The listing builds one solid part. Answer for the finished solid, in the listing's coordinates (mm). Face numbers are marked on the shaded views. A direction names the side the tool comes from. Coordinates: 2 decimals unless noted, no trailing zeros. Order: outer loops, then holes, each group sorted by start corner. A loop starts at its lowest first (then second) coordinate and runs counter-clockwise, first axis right, second up. Notation, with made-up numbers: (52.25, -4.5) -> (94.25, -4.5) arc R23 cw to (94.25, 29.5) -> close; hole circle Ø3 at (-28.5, 26.25). An arc over 180 degrees is marked (long way). Return JSON: item names as keys, results as strings.
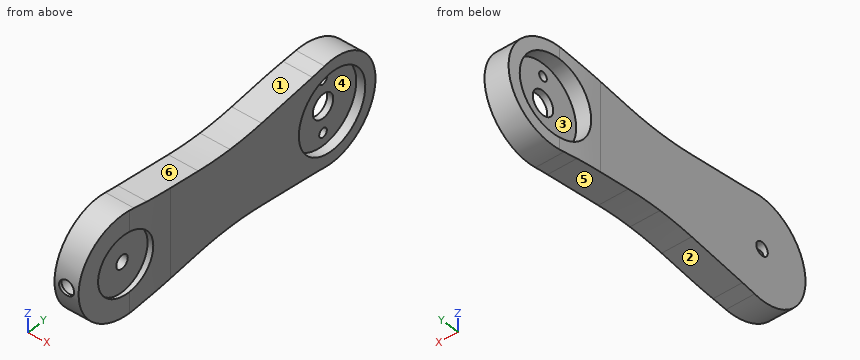
```python
from build123d import *

# Parameters (mm, degrees)
SALIENTE_EXTRUIR1_DEPTH     = 10
CROQUIS3_R                  = 10
CORTAR_EXTRUIR1_DEPTH       = 2
CORTAR_EXTRUIR5_START       = -10
CROQUIS7_R                  = 2.25
CORTAR_EXTRUIR5_DEPTH       = 55.115174372
CROQUIS8_R                  = 2.5
CORTAR_EXTRUIR6_DEPTH       = 19
CORTAR_EXTRUIR19_START      = -11
CROQUIS12_R                 = 3.5
CORTAR_EXTRUIR19_DEPTH      = 5
CORTAR_EXTRUIR20_DEPTH      = 99.634499619
CORTAR_EXTRUIR20_DEPTH_BACK = 99.634499619
CROQUIS13_R                 = 4
CROQUIS13_R_2               = 1.5
CROQUIS17_R                 = 13
CORTAR_EXTRUIR22_DEPTH      = 5
CORTAR_EXTRUIR23_START      = -3
CROQUIS15_R                 = 13
CORTAR_EXTRUIR23_DEPTH      = 3
CORTAR_EXTRUIR24_DEPTH      = 99.816823039
CORTAR_EXTRUIR24_DEPTH_BACK = 99.816823039
CROQUIS18_OUTSIDE_W         = 35.844
CROQUIS18_OUTSIDE_H         = 139.673


with BuildPart() as part:
    # Croquis1 → Saliente-Extruir1 (new body)
    with BuildSketch(Plane(origin=(0, 0, 0), x_dir=(0, 0, -1), z_dir=(1, 0, 0))):
        with BuildLine():
            Line((-16.039395606, 7.658342494), (-13.557839382, 27.510792285))
            ThreePointArc((-13.557839382, 27.510792285), (-12.978866844, 33.700521588), (-12.785627053, 39.914265744))
            Line((-12.785627053, 39.914265744), (12.785627053, 39.914265744))
            ThreePointArc((12.785627053, 39.914265744), (12.978866844, 33.700521588), (13.557839382, 27.510792285))
            Line((13.557839382, 27.510792285), (16.039395606, 7.658342494))
            ThreePointArc((16.039395606, 7.658342494), (16.365368489, 5.282403528), (16.748223211, 2.914964711))
            ThreePointArc((16.748223211, 2.914964711), (0, -17), (-16.748223211, 2.914964711))
            ThreePointArc((-16.748223211, 2.914964711), (-16.365368489, 5.282403528), (-16.039395606, 7.658342494))
        make_face()
    saliente_extruir1 = extrude(amount=-SALIENTE_EXTRUIR1_DEPTH)

    # Croquis3 → Cortar-Extruir1 (cut)
    with BuildSketch(Plane(origin=(0, 0, 0), x_dir=(0, 0, -1), z_dir=(1, 0, 0))):
        Circle(CROQUIS3_R)
    cortar_extruir1 = extrude(amount=-CORTAR_EXTRUIR1_DEPTH, mode=Mode.SUBTRACT)

    # Croquis7 → Cortar-Extruir5 (cut)
    with BuildSketch(Plane(origin=(-2, 0, 0), x_dir=(0, 0, -1), z_dir=(1, 0, 0)).offset(CORTAR_EXTRUIR5_START)):
        with Locations(Location((0, 0, 0), (0, 0, 180))):
            Circle(CROQUIS7_R)
    cortar_extruir5 = extrude(amount=CORTAR_EXTRUIR5_DEPTH, mode=Mode.SUBTRACT)

    # Croquis8 → Cortar-Extruir6 (cut)
    with BuildSketch(Plane(origin=(0, 0, 0), x_dir=(1, 0, 0), z_dir=(0, 1, 0))):
        with Locations(Location((-6, 0, 0), (0, 0, 270))):
            Circle(CROQUIS8_R)
    extrude(amount=-CORTAR_EXTRUIR6_DEPTH, mode=Mode.SUBTRACT)

    # Croquis12 → Cortar-Extruir19 (cut)
    with BuildSketch(Plane(origin=(0, 0, 0), x_dir=(1, 0, 0), z_dir=(0, 1, 0)).offset(CORTAR_EXTRUIR19_START)):
        with Locations(Location((-6, 0, 0), (0, 0, 270))):
            Circle(CROQUIS12_R)
    extrude(amount=-CORTAR_EXTRUIR19_DEPTH, mode=Mode.SUBTRACT)

    # Simetría1: Saliente-Extruir1, Cortar-Extruir1, Cortar-Extruir5 across plane
    add(saliente_extruir1.mirror(Plane(origin=(-10, 39.914265744, 12.785627053), x_dir=(0, 0, 1), z_dir=(0, 1, 0))))
    add(cortar_extruir1.mirror(Plane(origin=(-10, 39.914265744, 12.785627053), x_dir=(0, 0, 1), z_dir=(0, 1, 0))), mode=Mode.SUBTRACT)
    add(cortar_extruir5.mirror(Plane(origin=(-10, 39.914265744, 12.785627053), x_dir=(0, 0, 1), z_dir=(0, 1, 0))), mode=Mode.SUBTRACT)

    # Croquis13 → Cortar-Extruir20 (cut, two sides: drawn at the far end of the back side and taken through both)
    with BuildSketch(Plane(origin=(-2, 0, 0), x_dir=(0, 0, -1), z_dir=(1, 0, 0)).offset(-CORTAR_EXTRUIR20_DEPTH_BACK)):
        with Locations((0, 79.828531488)):
            Circle(CROQUIS13_R)
        with Locations((8.75, 79.828531488)):
            Circle(CROQUIS13_R_2)
        with Locations((-8.75, 79.828531488)):
            Circle(CROQUIS13_R_2)
    extrude(amount=CORTAR_EXTRUIR20_DEPTH + CORTAR_EXTRUIR20_DEPTH_BACK, mode=Mode.SUBTRACT)

    # Croquis17 → Cortar-Extruir22 (cut)
    with BuildSketch(Plane.ZY.offset(10)):
        with Locations((0, 79.828531488)):
            Circle(CROQUIS17_R)
    extrude(amount=-CORTAR_EXTRUIR22_DEPTH, mode=Mode.SUBTRACT)

    # Croquis15 → Cortar-Extruir23 (cut)
    with BuildSketch(Plane(origin=(0, 0, 0), x_dir=(0, 0, -1), z_dir=(1, 0, 0)).offset(CORTAR_EXTRUIR23_START)):
        with Locations(Location((0, 79.828531488, 0), (0, 0, 180))):
            Circle(CROQUIS15_R)
    extrude(amount=CORTAR_EXTRUIR23_DEPTH, mode=Mode.SUBTRACT)

    # Croquis18 outside → Cortar-Extruir24 (cut, two sides: drawn at the far end of the back side and taken through both)
    with BuildSketch(Plane.XY.offset(-CORTAR_EXTRUIR24_DEPTH_BACK)):
        with Locations((-5, 39.9145)):
            Rectangle(CROQUIS18_OUTSIDE_W, CROQUIS18_OUTSIDE_H)
        with BuildLine():
            Line((-8, 96.828531488), (0, 96.828531488))
            Line((0, 96.828531488), (0, 16.62668343))
            ThreePointArc((0, 16.62668343), (-0.148203384, 8.928671381), (-0.592593895, 1.242068046))
            Line((-0.592593895, 1.242068046), (-2, -17))
            Line((-2, -17), (-10, -17))
            Line((-10, -17), (-10, 63.201848057))
            ThreePointArc((-10, 63.201848057), (-9.851796616, 70.899860107), (-9.407406105, 78.586463442))
            Line((-9.407406105, 78.586463442), (-8, 96.828531488))
        make_face(mode=Mode.SUBTRACT)
    extrude(amount=CORTAR_EXTRUIR24_DEPTH + CORTAR_EXTRUIR24_DEPTH_BACK, mode=Mode.SUBTRACT)


solid = part.part
```
Item 1: Flat-ended cylindrical pins translate along their axes: pin 1 (1.5 mm diameter, centred on x = -4.5, z = 1, fed in from -Y); pin 2 (4 mm diameter, centred on x = -6, z = 0, fed in from -Y); pin 3 (13 mm diameter, centred on y = 76, z = -5, fed in from +X). Find the tip coordinate at first contact, or state that the pin passes through.
Answer list:
{"pin 1": "y = -16.96", "pin 2": "y = 1.03", "pin 3": "x = -3"}
Item 2: The part is cut by section C-C on y = 89. Determine the outline of the cut face in (x, z).
Answer list:
{"outline": "(-8.6, -14.31) -> (0, -14.31) -> (0, -9.21) -> (-3, -9.21) -> (-3, 9.21) -> (0, 9.21) -> (0, 14.31) -> (-8.6, 14.31) -> (-8.6, 9.21) -> (-5, 9.21) -> (-5, -9.21) -> (-8.6, -9.21) -> close"}
Item 3: Determine the mould class of the marked faces 1, 2 and 3 for opening direction Z: pulls with the +Z half, pulls with the -Z half, needs draft (parallel to the pull), parting line crosses it, or undercut.
Answer list:
{"face 1": "pulls with the +Z half", "face 2": "pulls with the -Z half", "face 3": "undercut"}
Item 4: Find the intervals of material crossed by probe 1 along Z at (x, y) = (-0.25, 41); probe 2 along X at (y, z) = (2, -5.5); probe 3 along Y at (x, z) = (-0.85, 0), in increasing order.
Answer list:
{"probe 1": "-12.79 to 12.79", "probe 2": "-10 to -2", "probe 3": "10 to 66.83, 92.83 to 96.83"}
Item 5: The part is cut by section A-A on z = -8.75. Determine the outline of the cut face in (x, y), plus the area to 3 significant figures.
Answer list:
{"outline": "(-10, -14.58) -> (-1.81, -14.58) -> (-1.06, -4.84) -> (-2, -4.84) -> (-2, 4.84) -> (-0.35, 4.84) arc R200 ccw to (0, 16.63) -> (0, 70.21) -> (-3, 70.21) -> (-3, 78.33) -> (-5, 78.33) -> (-5, 70.21) -> (-9.88, 70.21) arc R200 ccw to (-10, 63.2) -> close; (-8.57, 89.44) -> (-5, 89.44) -> (-5, 81.33) -> (-3, 81.33) -> (-3, 89.44) -> (0, 89.44) -> (0, 94.4) -> (-8.19, 94.4) -> close", "area": "887 mm2"}
Item 6: The part is cut by section D-D on z = 1. Count the separate pieces of the cut face and the enclosed holes in it, plus the area to 3 significant figures.
Answer list:
{"separate pieces": "4", "enclosed holes": "0", "area": "744 mm2"}
Item 7: The part is cut by section B-B on x = -6. Determine the outline of the cut face in (y, z), plus the area to 3 significant figures.
Answer list:
{"outline": "(-16.82, -2.5) arc R17 ccw to (2.91, -16.75) arc R100 cw to (7.66, -16.04) -> (27.51, -13.56) arc R100 cw to (52.32, -13.56) -> (72.17, -16.04) arc R100 cw to (76.91, -16.75) arc R17 ccw (long way) to (76.91, 16.75) arc R100 cw to (72.17, 16.04) -> (52.32, 13.56) arc R100 cw to (27.51, 13.56) -> (7.66, 16.04) arc R100 cw to (2.91, 16.75) arc R17 ccw to (-16.82, 2.5) -> (-16, 2.5) -> (-16, 3.5) -> (-11, 3.5) -> (-11, 2.5) -> (0, 2.5) -> (0, 2.25) arc R2.25 cw to (0, -2.25) -> (0, -2.5) -> (-11, -2.5) -> (-11, -3.5) -> (-16, -3.5) -> (-16, -2.5) -> close; hole circle Ø26 at (79.83, 0)", "area": "2,600 mm2"}
Item 8: Which of the six approach directions +Z, -Z, +X, -X, +Y, -Y give full straight-line access (tool end or side, diameter ignored) to the marked faces 4, 5 and 6?
Answer list:
{"face 4": "+X", "face 5": "-Z, +X, -X", "face 6": "+Z, +X, -X"}
